Autodesk Inventor part; units mm, degrees
ref_plane "Work Plane2" through (-3.5, -134.0004, -5) normal (0, 0, -1) x (0, 1, 0)
ref_plane "YZ Plane" through (0, 0, 0) normal (1, 0, 0) x (0, 1, 0)
ref_plane "XZ Plane" through (0, 0, 0) normal (0, 1, 0) x (-1, 0, 0)
sketch "Sketch1" plane through (0, 0, 0) normal (1, 0, 0) x (0, 1, 0)
  line L0 (0, 0) -> (30, 0)
  line L1 (30, 0) -> (30, 20)
  line L2 (30, 20) -> (0, 20)
  line L3 (0, 20) -> (0, 0)
  dimension "d0" = 30
  dimension "d1" = 20
extrude "Extrusion1" add sketch "Sketch1" along normal blind 14
ref_plane "Work Plane1" through (7, 0, 0) normal (-1, 0, 0) x (0, 0, 1)
sketch "Sketch2" plane through (7, 0, 0) normal (-1, 0, 0) x (0, 0, 1)
  line L0 (20, 0) -> (0, 0)
  line L1 (10, 0) -> (10, 30)
  line L2 (0, 30) -> (20, 30)
  line L3 (3.8, 5.4) -> (16.2, 5.4)
  line L4 (16.2, 5.4) -> (16.2, 24.6)
  line L5 (16.2, 24.6) -> (3.8, 24.6)
  line L6 (3.8, 24.6) -> (3.8, 5.4)
  line L7 (3.8, 5.4) -> (16.2, 24.6) construction
  line L8 (16.2, 5.4) -> (3.8, 24.6) construction
  line L9 (10, 5.4) -> (6.5, 5.4)
  line L10 (6.5, 5.4) -> (6.5, 0)
  line L11 (6.5, 0) -> (10, 0)
  line L12 (10, 0) -> (10, 5.4)
  line L13 (10, 24.6) -> (6.5, 24.6)
  line L14 (6.5, 24.6) -> (6.5, 30)
  line L15 (6.5, 30) -> (10, 30)
  line L16 (10, 30) -> (10, 24.6)
  line L17 (10, 24.6) -> (3.8, 24.6)
  line L18 (3.8, 24.6) -> (3.8, 5.4)
  line L19 (3.8, 5.4) -> (10, 5.4)
  line L20 (10, 5.4) -> (10, 24.6)
  point P0 (10, 15)
  dimension "d5" = 12.4
  dimension "d6" = 19.2
  dimension "d7" = 3.5
revolve "Revolution1" cut sketch "Sketch2" angle 360 about axis through (7, 0, 10) along (0, 1, 0) contours L0 L10 L3 L1 | L3 L6 L5 L1 | L5 L14 L2 L1
sketch "Sketch3" plane through (0, 0, 20) normal (0, 0, 1) x (1, 0, 0)
  line L0 (0, 30) -> (0, 0)
  line L1 (0, 0) -> (14, 0)
  line L2 (14, 30) -> (14, 0)
  line L3 (0, 30) -> (14, 30)
  line L4 (0, 0) -> (0, 30)
  line L5 (0, 0) -> (-7, 0)
  line L6 (-7, 0) -> (-7, 30)
  line L7 (-7, 30) -> (0, 30)
  line L8 (0, 30) -> (0, 0)
  line L9 (0, 30) -> (14, 30)
  circle A0 centre (-3.1, 5) radius 3.1
  line L10 (0, 30) -> (0, 0)
  circle A1 centre (-3.1, 25) radius 3.1
  dimension "d9" = 7
  dimension "d10" = 6.2
  dimension "d11" = 6.2
  dimension "d12" = 5
  dimension "d13" = 5
extrude "Extrusion2" add sketch "Sketch3" against normal up to surface (20 mm away) contours L0 L5 L6 L7
sketch "Sketch4" plane through (-7, 0, 20) normal (-1, 0, 0) x (0, 0, 1)
  line L0 (-16.2, 24.6) -> (-16.2, 5.4)
  line L1 (-15, 24.5) -> (-5, 24.5)
  line L2 (-13.5, 24.6) -> (-6.5, 24.6)
  line L3 (-16.2, 5.4) -> (-3.8, 5.4)
  line L4 (-3.8, 24.6) -> (-3.8, 5.4)
  line L5 (-16.2, 24.6) -> (-3.8, 24.6)
  line L6 (-17, 25) -> (-3, 25)
  line L7 (-3, 25) -> (-3, 5)
  line L8 (-3, 5) -> (-17, 5)
  line L9 (-17, 5) -> (-17, 25)
  line L10 (-17, 25) -> (-3, 5) construction
  line L11 (-3, 25) -> (-17, 5) construction
  line L12 (-13.5, 30.2686) -> (-6.5, 30.2686)
  line L13 (-6.5, 30.2686) -> (-6.5, 25)
  line L14 (-6.5, 25) -> (-13.5, 25)
  line L15 (-13.5, 25) -> (-13.5, 30.2686)
  line L16 (-13.5, 30.2686) -> (-6.5, 25) construction
  line L17 (-6.5, 30.2686) -> (-13.5, 25) construction
  line L18 (-13.5, -0.71) -> (-6.5, -0.71)
  line L19 (-6.5, -0.71) -> (-6.5, 5)
  line L20 (-6.5, 5) -> (-13.5, 5)
  line L21 (-13.5, 5) -> (-13.5, -0.71)
  line L22 (-13.5, -0.71) -> (-6.5, 5) construction
  line L23 (-6.5, -0.71) -> (-13.5, 5) construction
  point P0 (-20, 0)
  point P1 (-10, 15)
  point P2 (-10, 27.6343)
  point P3 (-10, 2.145)
  dimension "d16" = 14
  dimension "d17" = 20
  dimension "d18" = 7
extrude "Extrusion3" cut sketch "Sketch4" against normal blind 13 contours L5 L2 L4 L3 L0 | L6 L7 L8 L9
sketch "Sketch5" plane through (14, 0, 0) normal (0, 0, -1) x (-1, 0, 0)
  line L0 (21, 30) -> (0, 30)
  line L1 (0, 0) -> (0, 30)
  line L2 (21, 0) -> (0, 0)
  line L3 (21, 30) -> (21, 0)
  circle A0 centre (17.1, 25) radius 3.1
  circle A1 centre (17.1, 5) radius 3.1
  point P0 (14, 0)
ref_plane "Work Plane2" through (-3.5, -134.0004, -5) normal (0, 0, -1) x (0, 1, 0)
extrude "Extrusion4" add sketch "Sketch5" along normal blind 12
sketch "Sketch6" plane through (-7, 0, 20) normal (-1, 0, 0) x (0, 0, 1)
  point P0 (-20, 0)
sketch "Sketch7" plane through (-7, 0, 20) normal (-1, 0, 0) x (0, 0, 1)
  line L0 (-3, 5) -> (-17, 5)
  line L1 (-17, 5) -> (-17, 25)
  line L2 (-17, 25) -> (-3, 25)
  line L3 (-3, 25) -> (-3, 5)
  line L4 (0, 0) -> (-32, 0)
  line L5 (0, 30) -> (0, 0)
  line L6 (0, 30) -> (-32, 30)
  line L7 (-32, 0) -> (-32, 30)
  circle A0 centre (-28, 10) radius 1.4
  circle A1 centre (-21, 20) radius 1.4
  point P0 (-20, 0)
  dimension "d23" = 2.8
  dimension "d24" = 2.8
  dimension "d25" = 10
  dimension "d26" = 10
  dimension "d27" = 4
  dimension "d28" = 4
extrude "Extrusion5" cut sketch "Sketch7" against normal through all contours A0 | A1
sketch "Sketch8" plane through (14, 0, 20) normal (0, 0, 1) x (1, 0, 0)
  line L0 (-10, 99.8613) -> (-10, -100.1387)
  line L1 (-4, 99.8613) -> (-4, -100.1387)
  circle A0 centre (-7, 15) radius 1.4
  line L2 (-21, 0) -> (0, 0)
  point P0 (-14, 0)
  dimension "d31" = 2.8
  dimension "d32" = 15
  dimension "d33" = 3
extrude "Extrusion6" cut sketch "Sketch8" against normal through all
properties part number "30_CUBE_openXY_slider"
Input: part model. Units: mm. Frame: model coordinates. A direction names the side the tool comes from. Coordinates: 2 decimals unless noted, no trailing zeros. Loops run counter-clockwise (first coordinate to the right, second up) from the corner with the lowest first, then second, coordinate; pieces in that order, holes last.
Q1. Section D-D, the plane x = 0.75. Return the cut outline in (y, z), and give its area (3 significant figures).
Results are:
outline: (0, -12) - (30, -12) - (30, 20) - (0, 20) - close; hole (5, 3) - (25, 3) - (25, 17) - (5, 17) - close; hole circle Ø2.8 at (10, -8); hole circle Ø2.8 at (20, -1)
area: 668 mm2
Q2. Mould query, pull axis X, two halves, no side actions, for faces 4 (the flat face through (6, 21.2, 16.4)), 5 (the cylindrical face through (10.47, 2.66, 10.46)), 6 (the flat face through (2, 5, 10)). Classes: +X half, -X half, draft (parallel to the pull), parting line (faces both ways), or undercut.
Results are:
face 4: -X half
face 5: undercut
face 6: draft
Q3. Section B-B, the plane z = -8. Return the cut outline in (x, y), and give its area (3 significant figures).
Results are:
outline: (-7, 0) - (14, 0) - (14, 8.6) - (-7, 8.6) - close; (-7, 11.4) - (14, 11.4) - (14, 30) - (-7, 30) - close; hole circle Ø6.2 at (-3.1, 5); hole circle Ø6.2 at (-3.1, 25); hole circle Ø2.8 at (7, 15)
area: 505 mm2
Q4. Section C-C, the plane y = 2.5. Return the cut outline in (x, z).
Results are:
outline: (-7, -12) - (-4.93, -12) - (-4.93, 20) - (-7, 20) - close; (-1.27, -12) - (14, -12) - (14, 20) - (-1.27, 20) - close; hole circle Ø7 at (7, 10)
Q5. Set-up query: faces 1 (the flat face through (6, 8.9, 16.4)), 2 (the cylindrical face through (13.2, 14.87, 9.85)), 3 (the flat face through (14, 15, 4)). Return all of +Z, -Z, +X, -X, +Y, -Y with unobstructed straight access to the full face (end or side cutting, diameter ignored); none if empty.
Results are:
face 1: -X
face 2: none
face 3: +Z, -Z, +X, +Y, -Y
Q6. Line query: line 1 along Z through (x, y) = (0.75, 23.5); line 2 along Z through (x, y) = (7, 3.9); line 3 along Y through (x, z) = (-3.1, -2.5). Output: solid intervals per line, ascending.
Results are:
line 1: z = -12 to 3, 17 to 20
line 2: z = -12 to 6.5, 13.5 to 20
line 3: y = 0 to 1.9, 8.1 to 21.9, 28.1 to 30
Q7. Contact query for a flat-ended pin moving along its axis: pin 1 (3 mm diameter, centred on y = 8, z = 5, fed in from -X). Output: stop coordinate, or through.
Results are:
pin 1: stops at x = 6
Q8. Section A-A, the plane x = 7. Return the cut outline in (y, z), and give its area (3 significant figures).
Results are:
outline: (0, -12) - (13.6, -12) - (13.6, 3.8) - (5.4, 3.8) - (5.4, 6.5) - (0, 6.5) - close; (0, 13.5) - (5.4, 13.5) - (5.4, 16.2) - (13.6, 16.2) - (13.6, 20) - (0, 20) - close; (16.4, -12) - (30, -12) - (30, 6.5) - (24.6, 6.5) - (24.6, 3.8) - (16.4, 3.8) - close; (16.4, 16.2) - (24.6, 16.2) - (24.6, 13.5) - (30, 13.5) - (30, 20) - (16.4, 20) - close; hole circle Ø2.8 at (10, -8); hole circle Ø2.8 at (20, -1)
area: 579 mm2
